Geometry check sheet. Reference: drawing and pictorial views, mm from the part's lowest x, y, z. Round coordinates to 2 decimals unless told otherwise and drop trailing zeros. Write each loop counter-clockwise with the first axis right and the second up, starting at its lowest first coordinate (ties: lowest second). Pieces come first, ordered by that corner, then holes. Notation, with made-up numbers: (-11, 21) -> (35, 21) arc R21 ccw to (35, 54) -> close; hole circle Ø3 at (-6.5, 33). An arc over 180 degrees is marked (long way). Answer as a JSON object with one key per item and string values. Group by question number.
(1) Sectioned sample at A-A on x = 90. Record the cut outline in (y, z).
(2) Sectioned sample at C-C on x = 105. Record the cut outline in (y, z), and give its area (3 significant figures).
(3) Draft check along Y on the marked faces 1 and 2. Enter one of: released by +Y, released by -Y, zero draft, split by the parting line, or undercut.
(4) Scan lines: L1, parallel to Z at x = 105, y = 4.1; L2, parallel to Z at x = 55, y = 3.45; L3, parallel to X at y = 2.6, z = 106. Record each from-to range of solid material in increasing order. Write a range as from..to.
(5) Sectioned sample at B-B on z = 55. Record the cut outline in (x, y).
(6) Sectioned sample at D-D on z = 5. Record the cut outline in (x, y), and give its area (3 significant figures).
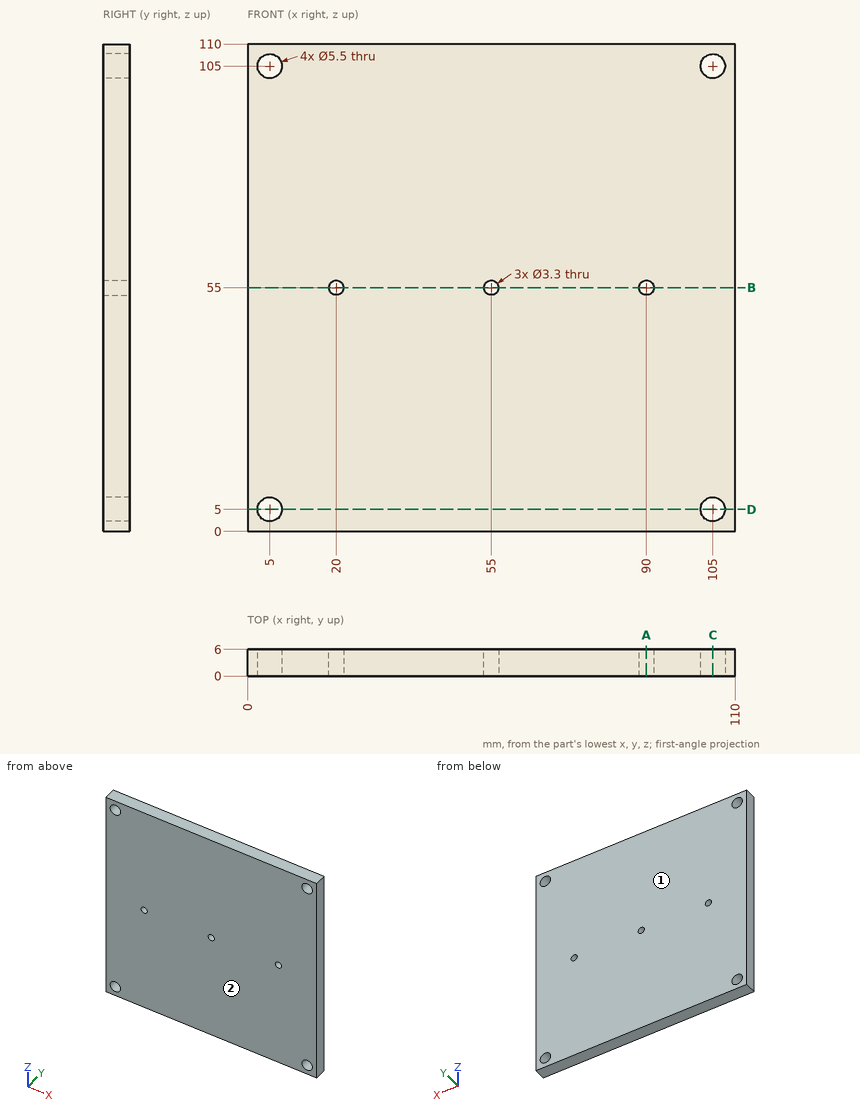
Computed values:
{
 "1": {"outline": "(0, 0) -> (6, 0) -> (6, 53.35) -> (0, 53.35) -> close; (0, 56.65) -> (6, 56.65) -> (6, 110) -> (0, 110) -> close"},
 "2": {"outline": "(0, 0) -> (6, 0) -> (6, 2.25) -> (0, 2.25) -> close; (0, 7.75) -> (6, 7.75) -> (6, 102.25) -> (0, 102.25) -> close; (0, 107.75) -> (6, 107.75) -> (6, 110) -> (0, 110) -> close", "area": "594 mm2"},
 "3": {"face 1": "released by +Y", "face 2": "released by -Y"},
 "4": {"L1": "0..2.25, 7.75..102.25, 107.75..110", "L2": "0..53.35, 56.65..110", "L3": "0..2.44, 7.56..102.44, 107.56..110"},
 "5": {"outline": "(0, 0) -> (18.35, 0) -> (18.35, 6) -> (0, 6) -> close; (21.65, 0) -> (53.35, 0) -> (53.35, 6) -> (21.65, 6) -> close; (56.65, 0) -> (88.35, 0) -> (88.35, 6) -> (56.65, 6) -> close; (91.65, 0) -> (110, 0) -> (110, 6) -> (91.65, 6) -> close"},
 "6": {"outline": "(0, 0) -> (2.25, 0) -> (2.25, 6) -> (0, 6) -> close; (7.75, 0) -> (102.25, 0) -> (102.25, 6) -> (7.75, 6) -> close; (107.75, 0) -> (110, 0) -> (110, 6) -> (107.75, 6) -> close", "area": "594 mm2"}
}
